Job drawing, mm, ordinate dimensions from the low corner. One solid piece. Give positions to 0.01 mm unless a question says otherwise; leave off trailing zeros. Write each loop counter-clockwise with the first axis right and the second up, starting at its lowest first coordinate (ties: lowest second). Pieces come first, ordered by that corner, then holes. Notation, with made-up numbers: M 66.25,63.5 L 111.25,63.5 A31 cw 111.25,91.5 Z; hole C 59.25,39.5 d6. An arc over 180 degrees is marked long. Use a Markdown table: item, result.
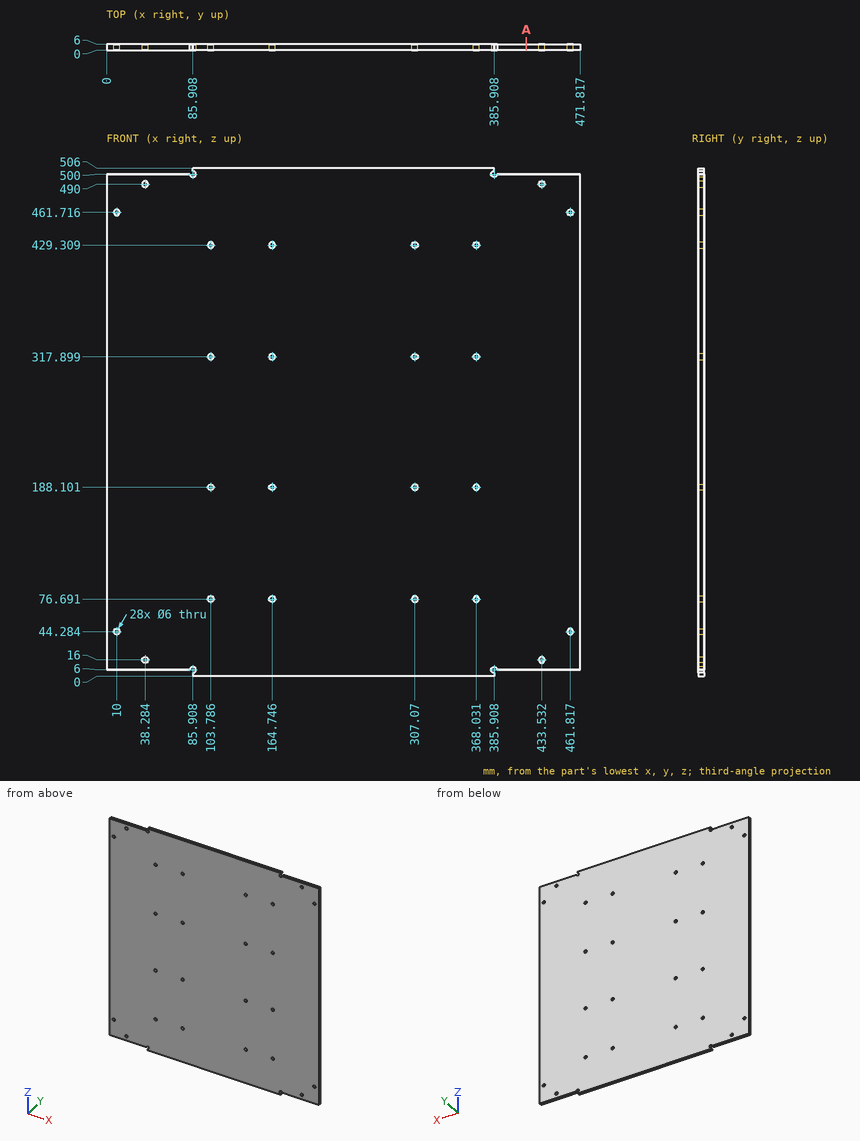
1. Cut at A-A, the plane x = 418. Give the cut face in (y, z).
Findings below:
| item | result |
|---|---|
| outline | M 0,6 L 6,6 L 6,500 L 0,500 Z |
2. Drill centre lines: L1, parallel to X at y = 2.8, z = 490 (1 decimal); L2, parallel to X at y = 0.7, z = 317.5 (1 decimal); L3, parallel to Z at x = 369.5, y = 0.45 (1 decimal). Where is each one in solid material? Low to high.
Findings below:
| item | result |
|---|---|
| L1 | 0 to 35.3, 41.3 to 430.5, 436.5 to 471.8 |
| L2 | 0 to 100.8, 106.8 to 161.8, 167.7 to 304.1, 310 to 365.1, 371 to 471.8 |
| L3 | 0 to 74.1, 79.3 to 185.5, 190.7 to 315.3, 320.5 to 426.7, 431.9 to 506 |
3. Drop flat-ended pins along their axis: P1, Ø7, axis at x = 10, z = 461.72, coming from the +Y side; P2, Ø0.9, axis at y = 4.5, z = 1, coming from the +X side. Give the stop position or say it passes through.
Findings below:
| item | result |
|---|---|
| P1 | y = 6 |
| P2 | x = 385.91 |
